Input: part model. Units: mm. Frame: model coordinates. A direction names the side the tool comes from. Round coordinates to 2 decimals unless told otherwise and drop trailing zeros. Order: outer loops, then holes, each group sorted by start corner. A loop starts at its lowest first (then second) coordinate and runs counter-clockwise, first axis right, second up. Notation, with made-up numbers: (-17.75, 76) - (4.25, 76) arc R22 ccw to (4.25, 87) - close; hole circle Ø6 at (31, 9.5). An arc over 180 degrees is marked (long way). One line per item, written item: value. Start each with the question number.
from build123d import *

# Parameters (mm, degrees)
F0_W     = 30
F0_H     = 30
F1_DEPTH = 10
F3_DEPTH = 20
F4_W     = 10
F4_H     = 15
F5_DEPTH = 30.001


with BuildPart() as f1:
    # F0 (on Front) → F1 (new body)
    with BuildSketch(Plane.XZ):
        with Locations((15, 15)):
            Rectangle(F0_W, F0_H)
    extrude(amount=F1_DEPTH)

    # F2 (on face) → F3 (join)
    with BuildSketch(Plane.XZ.offset(10)):
        Polygon((0, 30), (0, 0), (30, 0), align=None)
    extrude(amount=F3_DEPTH)

    # F4 (on face) → F5 (cut, through all)
    with BuildSketch(Plane(origin=(0, 0, 0), x_dir=(0, -1, 0), z_dir=(-1, 0, 0))):
        with Locations((15, 22.5)):
            Rectangle(F4_W, F4_H)
    extrude(amount=-F5_DEPTH, mode=Mode.SUBTRACT)


solid = f1.part
1. Section B-B (x = 9.5). Return the cut outline in (y, z).
2. Set-up query: faces 1 (the face through (0, -15, 12)), 2 (the face through (18, -10, 21)), 3 (the face through (6, -20, 21)), 4 (the face through (19, -22, 11)). Return all of +Z, -Z, +X, -X, +Y, -Y with unobstructed straight access to the full face (end or side cutting, diameter ignored); none if empty.
3. Line query: line 1 (Y direction, x = 13, z = 22); line 2 (Z direction, x = 11.5, y = -10.25); line 3 (Y direction, x = 6.5, z = 15.5). Output: solid intervals per line, ascending. Write a range as from..to.
4. Pull-direction query (Y, two-part tool) for faces 5 (the face through (15, -15, 0)), 6 (the face through (8, -30, 9)), 7 (the face through (7, -15, 15)); classes: released by +Y, released by -Y, zero draft, split by the parting line, or undercut.
5. Section C-C (z = 8.5). Return the cut outline in (x, y).
6. Section A-A (z = 25). Return the cut outline in (x, y).
7. Pin query (flat end, axial travel): pin 1 (2 mm diameter, centred on x = 24.5, z = 19.5, fed in from -Y); pin 2 (1.5 mm diameter, centred on y = -24.5, z = 5, fed in from +X); pin 3 (5 mm diameter, centred on y = -26, z = 21, fed in from +X). Return the tip coordinate at first contact, or that it passes through.
8. Section D-D (y = -17.75). Return the cut outline in (x, z).
Solved:
1. outline: (-30, 0) - (0, 0) - (0, 30) - (-10, 30) - (-10, 15) - (-20, 15) - (-20, 20.5) - (-30, 20.5) - close
2. face 1: +Z, -Z, -X, +Y, -Y
2. face 2: +Z, +X
2. face 3: +Z, +X, -X
2. face 4: +Z, +X, -Y
3. line 1: y = -10..0
3. line 2: z = 0..15
3. line 3: y = -30..-20, -10..0
4. face 5: zero draft
4. face 6: released by -Y
4. face 7: undercut
5. outline: (0, -30) - (21.5, -30) - (21.5, -10) - (30, -10) - (30, 0) - (0, 0) - close
6. outline: (0, -30) - (5, -30) - (5, -20) - (0, -20) - close; (0, -10) - (30, -10) - (30, 0) - (0, 0) - close
7. pin 1: stops at y = -10
7. pin 2: stops at x = 25.75
7. pin 3: stops at x = 11.5
8. outline: (0, 0) - (30, 0) - (15, 15) - (0, 15) - close
